from build123d import *
from build123d.topology import SkipClean

# Parameters (mm, degrees)
CROQUIS1_R                   = 4
SALIENTE_EXTRUIR1_DEPTH      = 12
SALIENTE_EXTRUIR2_DEPTH      = 14
SALIENTE_EXTRUIR2_DEPTH_BACK = 25


with BuildPart() as part:
    # Croquis1 → Saliente-Extruir1 (new body)
    with BuildSketch(Plane(origin=(0, 0, 0), x_dir=(1, 0, 0), z_dir=(0, 1, 0))):
        with Locations(Location((0, 0, 0), (0, 0, 270))):
            Circle(CROQUIS1_R)
    extrude(amount=SALIENTE_EXTRUIR1_DEPTH)

    # Croquis2 → Saliente-Extruir2 (add, two sides: drawn at the far end of the back side and taken through both)
    with SkipClean():  # the faces are left unmerged after this step: merging them gives an invalid solid
        with BuildSketch(Plane(origin=(0, 12, 0), x_dir=(1, 0, 0), z_dir=(0, 1, 0)).offset(-SALIENTE_EXTRUIR2_DEPTH_BACK)):
            with BuildLine():
                Line((-2.645751311, -3), (2.645751311, -3))
                ThreePointArc((2.645751311, -3), (4, 0), (2.645751311, 3))
                Line((2.645751311, 3), (-2.645751311, 3))
                ThreePointArc((-2.645751311, 3), (-4, 0), (-2.645751311, -3))
            make_face()
        extrude(amount=SALIENTE_EXTRUIR2_DEPTH + SALIENTE_EXTRUIR2_DEPTH_BACK)


solid = part.part
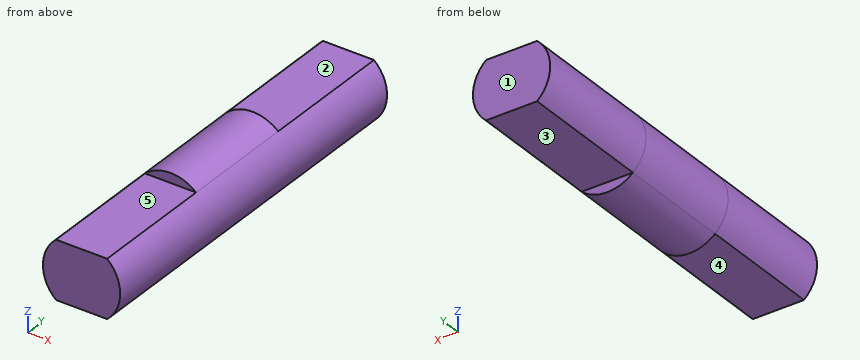
Read the model definition and answer for the solid it produces. Units are mm, in the model's axes. Face numbers are marked on the shaded views. A direction names the side the tool comes from. Give positions to 0.01 mm unless a question says otherwise; leave off trailing zeros. Write each loop counter-clockwise with the first axis right and the second up, starting at its lowest first coordinate (ties: lowest second). Pieces come first, ordered by that corner, then holes. Notation, with made-up numbers: (30, 50.25) - (79, 50.25) arc R25 ccw to (79, 87.25) - close; hole circle Ø4 at (12, 76). An arc over 180 degrees is marked (long way). Use CSV: the item, a comma, the result in double quotes. Start each with the question number.
Item 1: The part is cut by section A-A, the plane x = 2.25. Give the vertices of the cut face in (y, z).
Item 2: For the marked faces 1, 2, 3, 4 and 5, determine the directions among +Z, -Z, +X, -X, +Y, -Y from which every point of the face is accessible in a straight line to the end or side of a thin tool.
Item 3: The part is cut by section C-C, the plane z = 1.5. Give the vertices of the cut face in (x, y), and give its area (3 significant figures).
Item 4: The part is cut by section D-D, the plane x = -1.25. Give the vertices of the cut face in (y, z), and give its area (3 significant figures).
Item 5: The part is cut by section B-B, the plane y = 5.5. Give the vertices of the cut face in (x, z).
Item 6: Consider line 1 (Z direction, x = -1.25, y = 22.5); line 2 (Y direction, x = -1.75, z = -3.5); line 3 (Z direction, x = 3, y = -4.5). Determine where each line is inside the solid, lowest interval first.
Item 7: Flat-ended cylindrical pins translate along their axes: P1, Ø4, axis at x = 1, y = 16.5, coming from the +Z side; P2, Ø1.6, axis at x = -0.5, y = 17.5, coming from the -Z side; P3, Ø2, axis at y = 6.5, z = -2, coming from the +X side. Find the tip coordinate at first contact, or state that the pin passes through.
Taken from the geometry:
1,outline,"(-13, -3) - (0, -3) - (0, -3.31) - (12, -3.31) - (12, -3) - (26, -3) - (26, 3) - (12, 3) - (12, 3.31) - (0, 3.31) - (0, 3) - (-13, 3) - close"
2,face 1,"+Z, -Z, +X, -X, +Y"
2,face 2,"+Z, +X, -X, +Y"
2,face 3,"-Z, +X, -X, +Y"
2,face 4,"-Z, +X, -X, -Y"
2,face 5,"+Z, +X, -X, -Y"
3,outline,"(-3.71, -13) - (3.71, -13) - (3.71, 26) - (-3.71, 26) - close"
3,area,"289 mm2"
4,outline,"(-13, -3) - (0, -3) - (0, -3.8) - (12, -3.8) - (12, -3) - (26, -3) - (26, 3) - (12, 3) - (12, 3.8) - (0, 3.8) - (0, 3) - (-13, 3) - close"
4,area,"253 mm2"
5,outline,"circle Ø8 at (0, 0)"
6,line 1,"-3 to 3"
6,line 2,"0 to 12"
6,line 3,"-2.65 to 2.65"
7,P1,"z = 3"
7,P2,"z = -3"
7,P3,"x = 3.87"
